Autodesk Fusion 360 part; units mm, degrees
sketch "Sketch1" plane through (0, 0, 0) normal (0, 0, 1) x (1, 0, 0)
  circle A0 centre (0, 0) radius 5.375
  line L0 (0, 0) -> (0, 45)
  line L1 (0, 0) -> (55, 0)
  line L2 (-15, -11) -> (15, -11)
  line L3 (15, -11) -> (15, 11)
  line L4 (15, 11) -> (-15, 11)
  line L5 (-15, 11) -> (-15, -11)
  circle A1 centre (0, 8) radius 1.5
  circle A2 centre (-8, 0) radius 1.5
  circle A3 centre (0, -8) radius 1.5
  circle A4 centre (8, 0) radius 1.5
  dimension "d5" = 10.75
  dimension "d9" = 3
  dimension "d10" = 8
  dimension "d12" = 360
  dimension "d14" = 3
  dimension "d27" = 30
extrude "Extrude1" add sketch "Sketch1" along normal blind 32.25 contours A0 L0 L1 L2 L3 L4 L5 A1 A4 | A0 L0 L1 L3 L4 A1 A4
sketch "Sketch2" plane through (15, 0, 0) normal (1, 0, 0) x (0, 0, -1)
  line L0 (0, -11) -> (0, 11)
  line L1 (0, 11) -> (-32.25, 11)
  line L2 (-32.25, 11) -> (-32.25, -11)
  line L3 (-32.25, -11) -> (0, -11)
  circle A0 centre (-32.25, 26) radius 4.25
  circle A1 centre (-32.25, 26) radius 15
  line L4 (0, 11) -> (0, 21.7299)
  line L5 (0, 21.7299) -> (-23.6464, 38.2873)
  dimension "d20" = 8.5
  dimension "d21" = 15
  dimension "d28" = 30
  dimension "d34" = 125
extrude "Extrude2" add sketch "Sketch2" against normal blind 5 contours L1 A1 L4 L5 | A1
ref_plane "WorkPlane1" through (0, 16.75, 24.9478) normal (1, 0, 0) x (0, 1, 0)
mirror "Mirror1" about plane through (0, 16.75, 24.9478) normal (1, 0, 0) of "Extrude2"
fillet "Fillet1" radius 5 2 edges at (-12.5, 11, 32.25) (12.5, 11, 32.25)
fillet "Fillet2" radius 2 1 edges at (-10, 8.8175, 32.25)
equation "Screw_Nut_Dia = 10 mm"
equation "Screw_Nut_bolt_Dia = 3 mm"
equation "Screw_Nut_Bolt_Pattern = 16 mm"
equation "d5 = Screw_Nut_Dia + 0.75 mm"
equation "d9 = Screw_Nut_bolt_Dia"
equation "d10 = Screw_Nut_Bolt_Pattern / 2"
equation "d13 = Screw_Nut_bolt_Dia"
equation "d14 = d13"
equation "d28 = 22 mm + 8 mm"
equation "d34 = 180 deg - 55 deg"
Geometry check sheet. Reference: the model listing, model coordinates, mm. A direction names the side the tool comes from. Give positions to 0.01 mm unless a question says otherwise; leave off trailing zeros. Loops run counter-clockwise (first coordinate to the right, second up) from the corner with the lowest first, then second, coordinate; pieces in that order, holes last. Notation, with made-up numbers: M 55,74 L 104,74 A25 cw 104,104 Z; hole C -40,-7.5 d6. An arc over 180 degrees is marked long. Write item = value, one per line. Start each with the question number.
1. Section check A-A, the plane x = 8. Enter the section's corners in (y, z).
2. Go/stop test with flat-tipped pins: P1, Ø1, axis at x = -4.5, y = 9.5, coming from the +Z side; P2, Ø2, axis at x = 11.5, y = 18.5, coming from the +Z side; P3, Ø16, axis at x = -3.5, z = 24, coming from the +Y side (3 decimals). Record where each tip stops, or that it passes through.
3. Draft check along Y on faces 5 (the face through (0, -11, 16)), 6 (the face through (0, 6, 0)), 7 (the face through (-0.7, -5.33, 15.9)). Enter one of: +Y half, -Y half, draft (parallel to the pull), parting line (faces both ways), or undercut.
4. Tool access check on faces 1 (the face through (-9.165, 9.757, 32.624)), 2 (the face through (-12.535, 31.942, 46.023)), 3 (the face through (3, -5, 32.25)), 4 (the face through (-10, 23, 23)). Record the directions out of +Z, -Z, +X, -X, +Y, -Y that give a thin tool (end or side, any length) a straight path to the whole face; none if there is none.
5. Section check C-C, the plane z = 39. Enter the section's corners in (x, y), plus the area to 3 significant figures.
6. Thickness scan on probe 1 along Y at (x, z) = (0, 24.5) (3 decimals); probe 2 along X at (y, z) = (15, 11.5); probe 3 along Y at (x, z) = (-8, 14). Record the ranges inside material, lowest first.
7. Section check B-B, the plane y = 0. Enter the section's corners in (x, z) (3 decimals), plus the area to 3 significant figures.
8. Section check D-D, the plane y = 8. Enter the section's corners in (x, z).
Values follow:
q1.outline = M -11,0 L -1.5,0 L -1.5,32.25 L -11,32.25 Z; M 1.5,0 L 11,0 L 11,32.25 L 1.5,32.25 Z
q2.P1 = 32.25
q2.P2 = 45.77
q2.P3 = 40.565
q3.face_5 = -Y half
q3.face_6 = draft
q3.face_7 = undercut
q4.face_1 = +Z, +Y, -Y
q4.face_2 = +X, -X
q4.face_3 = +Z, -Y
q4.face_4 = +Z, -Z, +Y
q5.outline = M -15,12.6 L -10,12.6 L -10,39.4 L -15,39.4 Z; M 10,12.6 L 15,12.6 L 15,39.4 L 10,39.4 Z
q5.area = 268 mm^2
q6.probe_1 = -11 to -9.5, -6.5 to -5.375, 5.375 to 6.5, 9.5 to 11
q6.probe_2 = -15 to -10, 10 to 15
q6.probe_3 = -11 to -1.5, 1.5 to 11
q7.outline = M -15,0 L -9.5,0 L -9.5,32.25 L -15,32.25 Z; M -6.5,0 L -5.375,0 L -5.375,32.25 L -6.5,32.25 Z; M 5.375,0 L 6.5,0 L 6.5,32.25 L 5.375,32.25 Z; M 9.5,0 L 15,0 L 15,32.25 L 9.5,32.25 Z
q7.area = 427 mm^2
q8.outline = M -15,0 L -1.5,0 L -1.5,32.25 L -8,32.25 A2 cw -8.85,32.44 L -15,32.44 Z; M 1.5,0 L 15,0 L 15,32.44 L 10,32.44 L 10,32.25 L 1.5,32.25 Z
